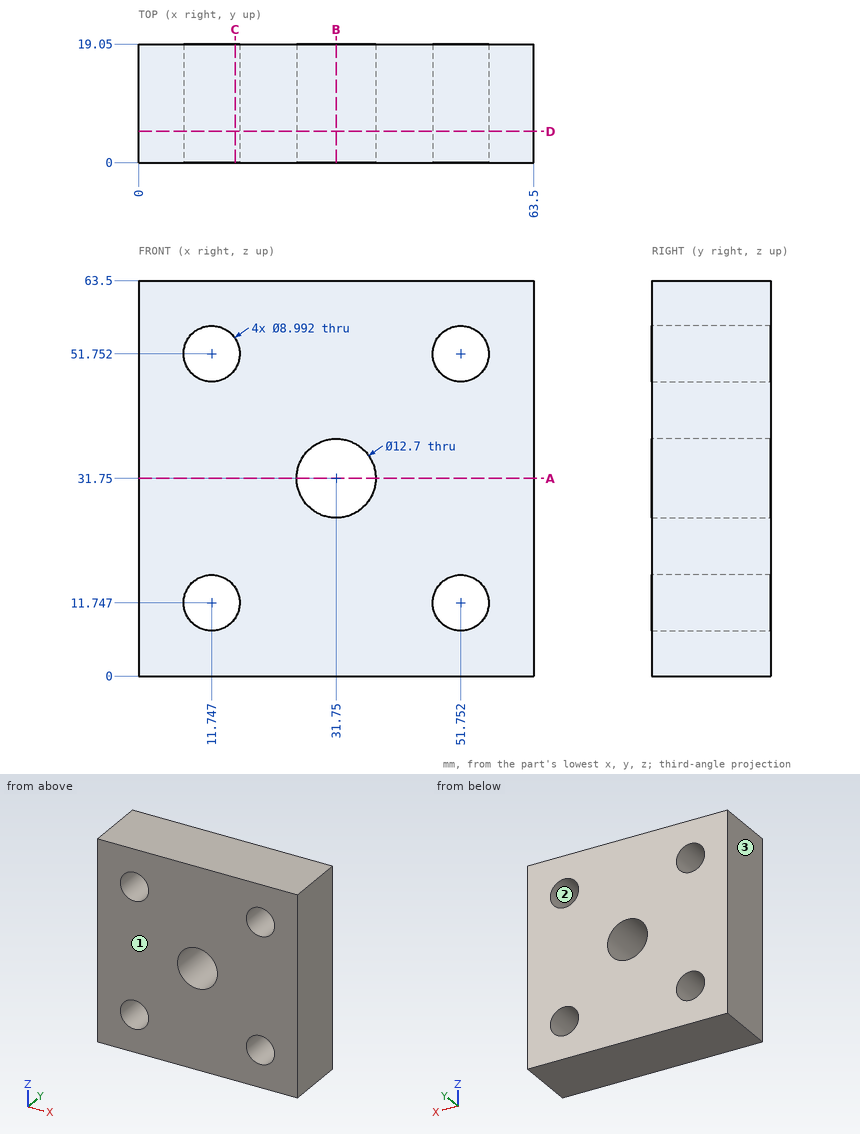
Design review of the part shown in the three views and the two pictorial views. Dimensions are in mm from the part's minimum x, y and z. Coordinates: 2 decimals unless noted, no trailing zeros. Loops run counter-clockwise (first coordinate to the right, second up) from the corner with the lowest first, then second, coordinate; pieces in that order, holes last. Notation, with made-up numbers: M 86,21 L 108,21 A16 cw 108,50 Z; hole C 80.25,79 d1. An arc over 180 degrees is marked long. Put each result on its own line as item: value. Start each with the question number.
Q1. Add section A-A (z = 31.75). Write out the cut boundary in (x, y), and give its area (3 significant figures).
Q2. Add section B-B (x = 31.75). Write out the cut boundary in (y, z), and give its area (3 significant figures).
Q3. Wall thickness on line 1 (X direction, y = 10.25, z = 12); line 2 (Z direction, x = 31.75, y = 6); line 3 (Z direction, x = 50, y = 5.75): over which ranges is each line inside the solid? List them lowest first.
Q4. Add section D-D (y = 5). Count the separate pieces of the cut face and the enclosed holes in it, and give its area (3 significant figures).
Q5. Clearance check with a flat-ended pin moving along its axis: pin 1 (11.5 mm diameter, centred on x = 51.75, z = 51.75, fed in from +Y). State where the tip first meets the part, or that it passes through.
Q6. The part is to be moulded in two halves that separate along X. For the marked faces 1, 2 and 3, say which applies: +X half, -X half, draft (parallel to the pull), parting line (faces both ways), or undercut.
Q7. Add section C-C (x = 15.5). Write out the cut boundary in (y, z), and give its area (3 significant figures).
Answers:
1. outline: M 0,0 L 25.4,0 L 25.4,19.05 L 0,19.05 Z; M 38.1,0 L 63.5,0 L 63.5,19.05 L 38.1,19.05 Z
1. area: 968 mm^2
2. outline: M 0,0 L 19.05,0 L 19.05,25.4 L 0,25.4 Z; M 0,38.1 L 19.05,38.1 L 19.05,63.5 L 0,63.5 Z
2. area: 968 mm^2
3. line 1: x = 0 to 7.26, 16.24 to 47.26, 56.24 to 63.5
3. line 2: z = 0 to 25.4, 38.1 to 63.5
3. line 3: z = 0 to 7.61, 15.89 to 47.61, 55.89 to 63.5
4. separate pieces: 1
4. enclosed holes: 5
4. area: 3,650 mm^2
5. pin 1: stops at y = 19.05
6. face 1: draft
6. face 2: undercut
6. face 3: -X half
7. outline: M 0,0 L 19.05,0 L 19.05,9.27 L 0,9.27 Z; M 0,14.22 L 19.05,14.22 L 19.05,49.28 L 0,49.28 Z; M 0,54.23 L 19.05,54.23 L 19.05,63.5 L 0,63.5 Z
7. area: 1,020 mm^2
